Can you work these out from the model? Positions are in its coordinate system, mm. Face numbers are marked on the shaded views. A direction names the side the tool comes from. Give positions to 0.01 mm unless a question says otherwise; leave off trailing zeros. Loops run counter-clockwise (first coordinate to the right, second up) from the corner with the lowest first, then second, coordinate; pieces in that order, holes last. Notation, with made-up numbers: (50, 14.25) - (96, 14.25) arc R14 cw to (96, 25.25) - close; hole circle Ø4 at (-6.5, -21.5). An arc over 180 degrees is marked (long way). Answer as a JSON object with one key per item and string values.
```python
from build123d import *

# Parameters (mm, degrees)
BOSS_EXTRU_2_DEPTH      = 18
ENL_V_MAT_EXTRU_1_DEPTH = 19
CONG_1_R                = 7
ESQUISSE3_R             = 6.5
ENL_V_MAT_EXTRU_2_DEPTH = 19


with BuildPart() as part:
    # Esquisse2 → Boss.-Extru.2 (new body)
    with BuildSketch(Plane.XY):
        with BuildLine():
            Line((0, 0), (60, 0))
            Line((60, 0), (60, 46.012238509))
            ThreePointArc((60, 46.012238509), (59.874827529, 46.793387794), (59.511844635, 47.496314371))
            ThreePointArc((59.511844635, 47.496314371), (60, 54), (66.503685629, 54.488155365))
            ThreePointArc((66.503685629, 54.488155365), (67.206612206, 54.125172471), (67.987761491, 54))
            Line((67.987761491, 54), (80, 54))
            Line((80, 54), (80, 94))
            Line((80, 94), (-20, 94))
            Line((-20, 94), (-20, 54))
            Line((-20, 54), (-7.987761491, 54))
            ThreePointArc((-7.987761491, 54), (-7.206612206, 54.125172471), (-6.503685629, 54.488155365))
            ThreePointArc((-6.503685629, 54.488155365), (0, 54), (0.488155365, 47.496314371))
            ThreePointArc((0.488155365, 47.496314371), (0.125172471, 46.793387794), (0, 46.012238509))
            Line((0, 46.012238509), (0, 0))
        make_face()
    extrude(amount=BOSS_EXTRU_2_DEPTH)

    # Esquisse1 → Enlèv. mat.-Extru.1 (cut, through all)
    with BuildSketch(Plane.XY):
        with BuildLine():
            Line((39.5, 28.248771852), (39.5, 25.751228148))
            ThreePointArc((39.5, 25.751228148), (39.599672829, 25.160561143), (39.88765279, 24.635309084))
            ThreePointArc((39.88765279, 24.635309084), (39.5, 18), (32.864690916, 17.61234721))
            ThreePointArc((32.864690916, 17.61234721), (32.339438857, 17.900327171), (31.748771852, 18))
            Line((31.748771852, 18), (28.251228148, 18))
            ThreePointArc((28.251228148, 18), (27.660561143, 17.900327171), (27.135309084, 17.61234721))
            ThreePointArc((27.135309084, 17.61234721), (20.5, 18), (20.11234721, 24.635309084))
            ThreePointArc((20.11234721, 24.635309084), (20.400327171, 25.160561143), (20.5, 25.751228148))
            Line((20.5, 25.751228148), (20.5, 28.248771852))
            ThreePointArc((20.5, 28.248771852), (20.400327171, 28.839438857), (20.11234721, 29.364690916))
            ThreePointArc((20.11234721, 29.364690916), (20.5, 36), (27.135309084, 36.38765279))
            ThreePointArc((27.135309084, 36.38765279), (27.660561143, 36.099672829), (28.251228148, 36))
            Line((28.251228148, 36), (31.748771852, 36))
            ThreePointArc((31.748771852, 36), (32.339438857, 36.099672829), (32.864690916, 36.38765279))
            ThreePointArc((32.864690916, 36.38765279), (39.5, 36), (39.88765279, 29.364690916))
            ThreePointArc((39.88765279, 29.364690916), (39.599672829, 28.839438857), (39.5, 28.248771852))
        make_face()
    extrude(amount=ENL_V_MAT_EXTRU_1_DEPTH, mode=Mode.SUBTRACT)

    # Congé1
    cong_1_edges = [part.edges().sort_by_distance(p)[0] for p in [
        (-20, 94, 9),
        (80, 94, 9),
        (60, 0, 9),
        (0, 0, 9),
    ]]
    fillet(cong_1_edges, radius=CONG_1_R)

    # Esquisse3 → Enlèv. mat.-Extru.2 (cut, through all)
    with BuildSketch(Plane.XY.offset(18)):
        with Locations((0, 74)):
            Circle(ESQUISSE3_R)
    extrude(amount=-ENL_V_MAT_EXTRU_2_DEPTH, mode=Mode.SUBTRACT)


solid = part.part
```
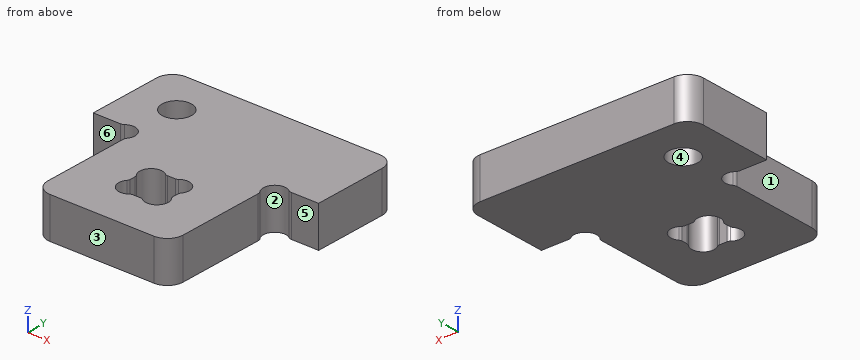
1) If we mould it in two halves opening along Y, with no side actions, what happens to the marked faces 1, 2 and 3? For each: released by +Y, released by -Y, zero draft, split by the parting line, or undercut.
Check sheet entries:
{"face 1": "zero draft", "face 2": "undercut", "face 3": "released by -Y"}
2) I need wall thicknesses on L1, parallel to X at y = 17, z = 7.5; L2, parallel to Y at x = 71, z = 2.75; L3, parallel to X at y = 21.5, z = 16. Which ranges of each line are inside material? Lowest first, please.
Check sheet entries:
{"L1": "0 to 21.93, 26.14 to 33.86, 38.07 to 60", "L2": "54 to 94", "L3": "0 to 19.04, 40.96 to 60"}
3) Imagine slicing it at A-A on y = 74. Write out the boundary of the cut face in (x, z), and give its area (3 significant figures).
Check sheet entries:
{"outline": "(-20, 0) - (-6.5, 0) - (-6.5, 18) - (-20, 18) - close; (6.5, 0) - (80, 0) - (80, 18) - (6.5, 18) - close", "area": "1,570 mm2"}
4) Imagine slicing it at C-C on y = 8.5. Write out the boundary of the cut face in (x, z).
Check sheet entries:
{"outline": "(0, 0) - (60, 0) - (60, 18) - (0, 18) - close"}
5) Imagine slicing it at B-B on z = 7.5. Give the number of separate pieces and of enclosed holes in the cut face, and give its area (3 significant figures).
Check sheet entries:
{"separate pieces": "1", "enclosed holes": "2", "area": "6,640 mm2"}
6) I'm going to push flat-ended pins straight in: P1, Ø9, axis at y = 20.5, z = 13, coming from the -X side; P2, Ø1.5, axis at x = 2, z = 12.5, coming from the -Y side; P3, Ø0.7, axis at y = 27.5, z = 12.5, coming from the +X side; P4, Ø11.5, axis at x = 0, y = 74, coming from the +Z side. Where does each tip first touch, or does it pass through?
Check sheet entries:
{"P1": "x = 0", "P2": "y = 1.44", "P3": "x = 60", "P4": "through"}
7) Which directions (+Z, -Z, +X, -X, +Y, -Y) give clear straight access to the entire face, cutting with the end or side of a thin tool? Please do the marked faces 4, 5 and 6.
Check sheet entries:
{"face 4": "+Z, -Z", "face 5": "+Z, -Z, +X, -Y", "face 6": "+Z, -Z, -X, -Y"}
